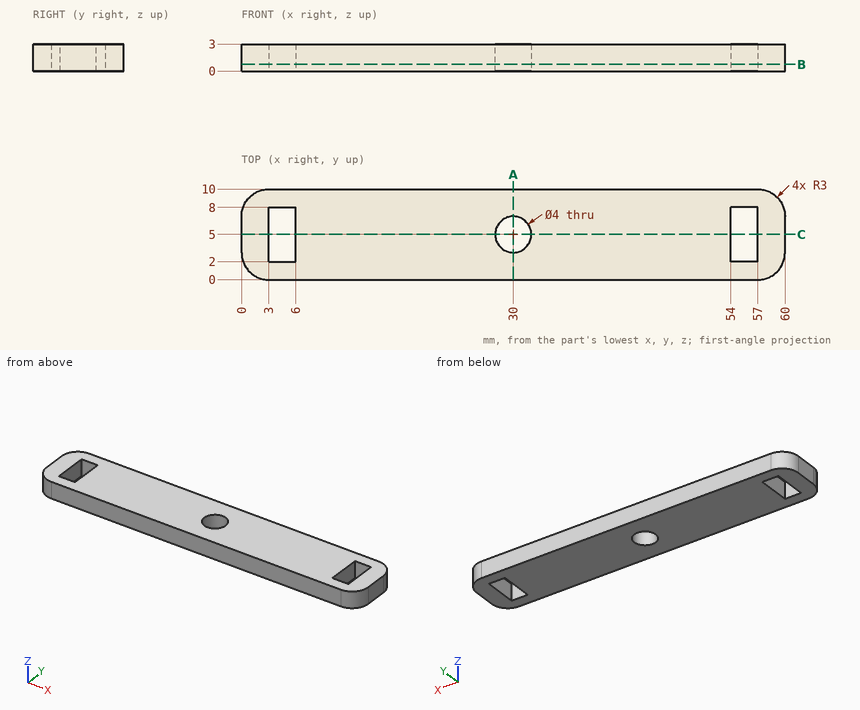
Can you work these out from the drawing? Everything is in mm from the part's minimum corner. Round coordinates to 2 decimals unless told otherwise and drop trailing zeros. Loops run counter-clockwise (first coordinate to the right, second up) from the corner with the lowest first, then second, coordinate; pieces in that order, holes last. Notation, with made-up numbers: (-28.5, 34.25) - (-10.5, 34.25) arc R21 cw to (-10.5, 71.25) - close; hole circle Ø2 at (-15.5, -24.5). An arc over 180 degrees is marked (long way). Answer in a Markdown table with one row per item. Add a question column.
(1) If we section it at B-B (z = 0.75): Please give me the cut outline in (x, y), plus the area to 3 significant figures.
(2) I'm going to push a flat-ended pin straight in: pin 1 (6 mm diameter, centred on x = 8, y = 3.5, fed in from -Z). Where does the tip first touch, or does it pass through?
(3) I need wall thicknesses on line 1 along Y through (x, z) = (30, 0.75); line 2 along X through (y, z) = (5.25, 0.2); line 3 along Y through (x, z) = (5, 2.35). Which ranges of each line are inside material? Lowest first, please.
(4) If we section it at C-C (y = 5): Please give me the cut outline in (x, z).
(5) If we section it at A-A (x = 30): Please give me the cut outline in (y, z), plus the area to 3 significant figures.
Model answer:
| question | item | result |
|---|---|---|
| 1 | outline | (0, 3) arc R3 ccw to (3, 0) - (57, 0) arc R3 ccw to (60, 3) - (60, 7) arc R3 ccw to (57, 10) - (3, 10) arc R3 ccw to (0, 7) - close; hole (3, 2) - (6, 2) - (6, 8) - (3, 8) - close; hole circle Ø4 at (30, 5); hole (54, 2) - (57, 2) - (57, 8) - (54, 8) - close |
| 1 | area | 544 mm² |
| 2 | pin 1 | stops at z = 0 |
| 3 | line 1 | y = 0 to 3, 7 to 10 |
| 3 | line 2 | x = 0 to 3, 6 to 28.02, 31.98 to 54, 57 to 60 |
| 3 | line 3 | y = 0 to 2, 8 to 10 |
| 4 | outline | (0, 0) - (3, 0) - (3, 3) - (0, 3) - close; (6, 0) - (28, 0) - (28, 3) - (6, 3) - close; (32, 0) - (54, 0) - (54, 3) - (32, 3) - close; (57, 0) - (60, 0) - (60, 3) - (57, 3) - close |
| 5 | outline | (0, 0) - (3, 0) - (3, 3) - (0, 3) - close; (7, 0) - (10, 0) - (10, 3) - (7, 3) - close |
| 5 | area | 18.0 mm² |
